Design review of the part built by this model. Coordinates are the model's own, in mm. Face numbers are marked on the shaded views. A direction names the side the tool comes from. Coordinates: 2 decimals unless noted, no trailing zeros. Write each loop counter-clockwise with the first axis right and the second up, starting at its lowest first coordinate (ties: lowest second). Pieces come first, ordered by that corner, then holes.
Q1. Add section B-B, the plane y = 9. Give the boundary of the cut face in (x, z), plus the area to 3 significant figures.
Q2. To check wall thickness, follow probe 1 along X at (y, z) = (9, 3); probe 2 along X at (y, z) = (-10.5, 2.75); probe 3 along Y at (x, z) = (-27, 8.25). State the ranges of each line that lie inside material, in increasing order.
Q3. Add section A-A, the plane x = -27. Give the boundary of the cut face in (y, z).
Q4. Add section D-D, the plane x = 12. Give the boundary of the cut face in (y, z), plus the area to 3 significant figures.
Q5. Clearance check with flat-ended pins moving along their axes: pin 1 Ø2 at (x, z) = (50.5, 5) entering from +Y; pin 2 Ø0.9 at (x, z) = (-22, 7) entering from +Y; pin 3 Ø10 at (x, y) = (50, 3) entering from -Z; pin 4 Ø4.5 at (y, z) = (-9, 5.5) entering from +X. State where each tip first meets the part, or that it passes through.
Q6. Add section C-C, the plane x = 45. Give the boundary of the cut face in (y, z).
Q7. Machinability: for the marked faces 1, 2 and 3, which of the approach directions +Z, -Z, +X, -X, +Y, -Y give a long, thin tool a straight path to every point of the face, cutting with its end or side? Answer none if there is none.
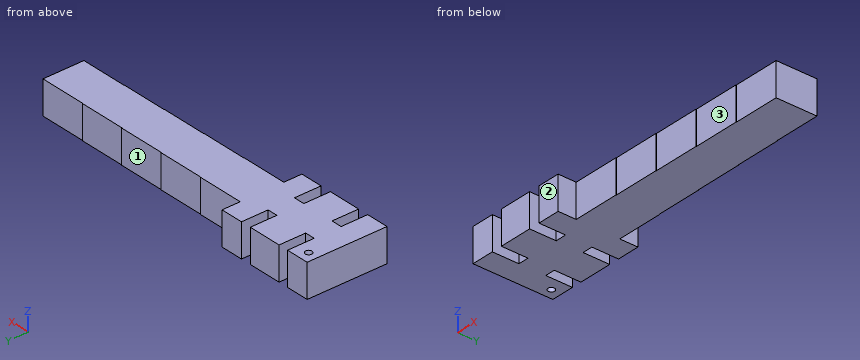
from build123d import *

# Parameters (mm, degrees)
GAUGE_BODY_DEPTH   = 5
NOTCH_3_0_SKETCH_W = 3
NOTCH_3_0_SKETCH_H = 9
NOTCH_3_0_DEPTH    = 6
NOTCH_3_1_SKETCH_W = 3.1
NOTCH_3_1_SKETCH_H = 9
NOTCH_3_1_DEPTH    = 6
NOTCH_3_2_SKETCH_W = 3.2
NOTCH_3_2_SKETCH_H = 9
NOTCH_3_2_DEPTH    = 6
NOTCH_3_3_SKETCH_W = 3.3
NOTCH_3_3_SKETCH_H = 9
NOTCH_3_3_DEPTH    = 6
MARK_HOLE_SKETCH_R = 1
MARK_HOLE_DEPTH    = 6


with BuildPart() as part:
    # gauge body sketch → gauge body (new, symmetric)
    with BuildSketch(Plane.XY.offset(5)):
        Polygon((-30, 12), (0, 12), (0, 6.55), (14, 6.55), (14, 6.45), (28, 6.45), (28, 6.35), (42, 6.35), (42, 6.25), (56, 6.25), (56, 6.15), (70, 6.15), (70, -6.15), (56, -6.15), (56, -6.25), (42, -6.25), (42, -6.35), (28, -6.35), (28, -6.45), (14, -6.45), (14, -6.55), (0, -6.55), (0, -12), (-30, -12), align=None)
    extrude(amount=GAUGE_BODY_DEPTH, both=True)

    # notch 3.0 sketch → notch 3.0 (cut, symmetric)
    with BuildSketch(Plane.XY.offset(5)):
        with Locations((-21.6, 8.5)):
            Rectangle(NOTCH_3_0_SKETCH_W, NOTCH_3_0_SKETCH_H)
    extrude(amount=NOTCH_3_0_DEPTH, both=True, mode=Mode.SUBTRACT)

    # notch 3.1 sketch → notch 3.1 (cut, symmetric)
    with BuildSketch(Plane.XY.offset(5)):
        with Locations((-8.4, 8.5)):
            Rectangle(NOTCH_3_1_SKETCH_W, NOTCH_3_1_SKETCH_H)
    extrude(amount=NOTCH_3_1_DEPTH, both=True, mode=Mode.SUBTRACT)

    # notch 3.2 sketch → notch 3.2 (cut, symmetric)
    with BuildSketch(Plane.XY.offset(5)):
        with Locations((-21.6, -8.5)):
            Rectangle(NOTCH_3_2_SKETCH_W, NOTCH_3_2_SKETCH_H)
    extrude(amount=NOTCH_3_2_DEPTH, both=True, mode=Mode.SUBTRACT)

    # notch 3.3 sketch → notch 3.3 (cut, symmetric)
    with BuildSketch(Plane.XY.offset(5)):
        with Locations((-8.4, -8.5)):
            Rectangle(NOTCH_3_3_SKETCH_W, NOTCH_3_3_SKETCH_H)
    extrude(amount=NOTCH_3_3_DEPTH, both=True, mode=Mode.SUBTRACT)

    # mark hole sketch → mark hole (cut, symmetric)
    with BuildSketch(Plane.XY.offset(5)):
        with Locations(Location((-27, 9, 0), (0, 0, 180))):
            Circle(MARK_HOLE_SKETCH_R)
    extrude(amount=MARK_HOLE_DEPTH, both=True, mode=Mode.SUBTRACT)


solid = part.part
Here are the results:
1. outline: (-30, 0) - (-28, 0) - (-28, 10) - (-30, 10) - close; (-26, 0) - (-23.1, 0) - (-23.1, 10) - (-26, 10) - close; (-20.1, 0) - (-9.95, 0) - (-9.95, 10) - (-20.1, 10) - close; (-6.85, 0) - (0, 0) - (0, 10) - (-6.85, 10) - close
1. area: 219 mm2
2. probe 1: x = -30 to -28, -26 to -23.1, -20.1 to -9.95, -6.85 to 0
2. probe 2: x = -30 to -23.2, -20 to -10.05, -6.75 to 0
2. probe 3: y = -12 to 8, 10 to 12
3. outline: (-12, 0) - (8, 0) - (8, 10) - (-12, 10) - close; (10, 0) - (12, 0) - (12, 10) - (10, 10) - close
4. outline: (-6.55, 0) - (6.55, 0) - (6.55, 10) - (-6.55, 10) - close
4. area: 131 mm2
5. pin 1: stops at y = 6.25
5. pin 2: stops at y = 4
5. pin 3: stops at z = 0
5. pin 4: stops at x = 0
6. outline: (-6.25, 0) - (6.25, 0) - (6.25, 10) - (-6.25, 10) - close
7. face 1: +Z, -Z, +X, +Y
7. face 2: +Z, -Z, +X, -X, -Y
7. face 3: +Z, -Z, +X, -Y
